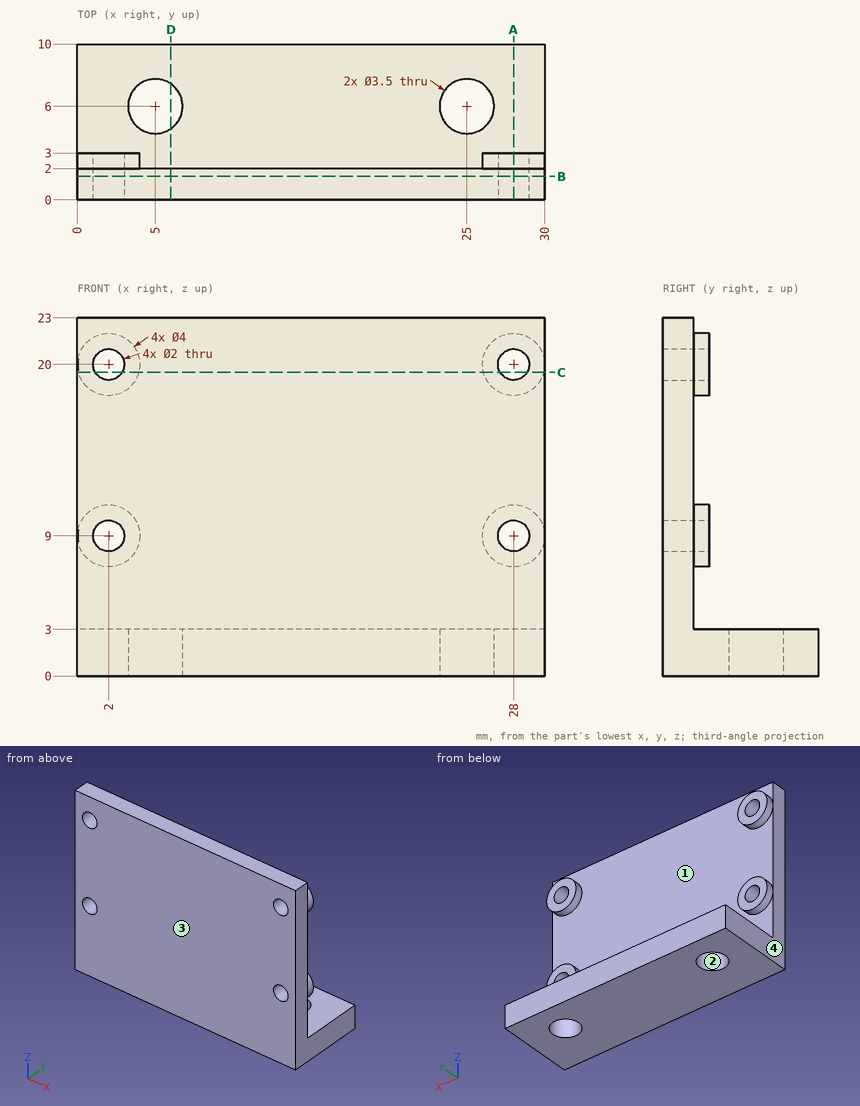
Here's the drawing with two shaded views (mm, measured from the low corner). I have some questions. Coordinates: 2 decimals unless noted, no trailing zeros. Write each loop counter-clockwise with the first axis right and the second up, starting at its lowest first coordinate (ties: lowest second). Pieces come first, ordered by that corner, then holes. Notation, with made-up numbers: (-9, -34.5) -> (25, -34.5) arc R8 cw to (25, -29.5) -> close; hole circle Ø7 at (12, 80). An arc over 180 degrees is marked (long way). One line per question, with ' | ' between items. Start each with the question number.
1. If we section it at C-C (z = 19.5): Please give me the cut outline in (x, y), and give its area (3 significant figures).
2. Thinking about a two-plate mould opening in Y: for the marked faces 1, 2, 3 and 4, which applies, pulls with the +Y half, pulls with the -Y half, needs draft (parallel to the pull), parting line crosses it, or undercut?
3. Please list where these lines run through material, in increasing order: line 1 along Z through (x, y) = (28, 1.55); line 2 along X through (y, z) = (1, 20); line 3 along Z through (x, y) = (28, 2.05).
4. Will these pins go through, and if not, where does the flat tip stop? P1, Ø3, axis at x = 18, y = 7.5, coming from the +Z side; P2, Ø1.2, axis at x = 2.5, z = 9.5, coming from the +Y side; P3, Ø2, axis at x = 13, z = 10, coming from the +Y side.
5. If we section it at B-B (y = 1.5): Please give me the cut outline in (x, z).
6. If we section it at A-A (x = 28): Please give me the cut outline in (y, z).
7. If we section it at D-D (x = 6): Please give me the cut outline in (y, z).
Return value:
1) outline: (0, 0) -> (1.13, 0) -> (1.13, 3) -> (0.06, 3) -> (0.06, 2) -> (0, 2) -> close; (2.87, 0) -> (27.13, 0) -> (27.13, 3) -> (26.06, 3) -> (26.06, 2) -> (3.94, 2) -> (3.94, 3) -> (2.87, 3) -> close; (28.87, 0) -> (30, 0) -> (30, 2) -> (29.94, 2) -> (29.94, 3) -> (28.87, 3) -> close | area: 57.4 mm²
2) face 1: pulls with the +Y half | face 2: undercut | face 3: pulls with the -Y half | face 4: needs draft
3) line 1: z = 0 to 8, 10 to 19, 21 to 23 | line 2: x = 0 to 1, 3 to 27, 29 to 30 | line 3: z = 0 to 3, 7 to 8, 10 to 11, 18 to 19, 21 to 22
4) P1: stops at z = 3 | P2: stops at y = 3 | P3: stops at y = 2
5) outline: (0, 0) -> (30, 0) -> (30, 23) -> (0, 23) -> close; hole circle Ø2 at (2, 9); hole circle Ø2 at (2, 20); hole circle Ø2 at (28, 9); hole circle Ø2 at (28, 20)
6) outline: (0, 0) -> (10, 0) -> (10, 3) -> (2, 3) -> (2, 7) -> (3, 7) -> (3, 8) -> (0, 8) -> close; (0, 10) -> (3, 10) -> (3, 11) -> (2, 11) -> (2, 18) -> (3, 18) -> (3, 19) -> (0, 19) -> close; (0, 21) -> (3, 21) -> (3, 22) -> (2, 22) -> (2, 23) -> (0, 23) -> close
7) outline: (0, 0) -> (4.56, 0) -> (4.56, 3) -> (2, 3) -> (2, 23) -> (0, 23) -> close; (7.44, 0) -> (10, 0) -> (10, 3) -> (7.44, 3) -> close
